from build123d import *

# Parameters (mm, degrees)
F0_W     = 82.55
F0_H     = 25.4
F1_DEPTH = 3.81
F2_W     = 2.54
F2_H     = 25.4
F3_DEPTH = 38.1
F4_R     = 7.62


with BuildPart() as f1:
    # F0 (on Top) → F1 (new body)
    with BuildSketch(Plane.XY):
        Rectangle(F0_W, F0_H)
    extrude(amount=F1_DEPTH)

    # F2 (on face) → F3 (join)
    with BuildSketch(Plane.XY.offset(3.81)):
        with Locations((-19.923125, 0)):
            Rectangle(F2_W, F2_H)
        with Locations((19.923125, 0)):
            Rectangle(F2_W, F2_H)
    extrude(amount=F3_DEPTH)

    # F4
    f4_edges = [f1.edges().sort_by_distance(p)[0] for p in [
        (-41.275, 12.7, 1.905),
        (-41.275, -12.7, 1.905),
        (41.275, 12.7, 1.905),
        (41.275, -12.7, 1.905),
        (-21.193125, 0, 3.81),
        (21.193125, 0, 3.81),
        (19.923125, 12.7, 41.91),
        (-19.923125, 12.7, 41.91),
        (-19.923125, -12.7, 41.91),
        (19.923125, -12.7, 41.91),
    ]]
    fillet(f4_edges, radius=F4_R)


solid = f1.part
Verification items for the finished model (mm, model axes). A direction names the side the tool comes from. Round coordinates to 2 decimals unless told otherwise and drop trailing zeros. Loops run counter-clockwise (first coordinate to the right, second up) from the corner with the lowest first, then second, coordinate; pieces in that order, holes last. Notation, with made-up numbers: (86.25, 49.5) - (96.25, 49.5) arc R18 cw to (96.25, 66.5) - close; hole circle Ø1 at (53.25, 8.5). An arc over 180 degrees is marked (long way). Answer in a Markdown table with one row per item. Add a question column.
Q1. Material ranges on line 1 (X direction, y = 2.25, z = 13); line 2 (Z direction, x = 12, y = -2.25); line 3 (X direction, y = -7.5, z = 6.5), recorded low to high.
Q2. Release check for a two-part mould opening along X. For faces 1 (the face through (-21.193, 0, 26)), 2 (the face through (18.653, 0, 23)), 3 (the face through (35, 0, 3.81)) record: pulls with the +X half, pulls with the -X half, needs draft (parallel to the pull), parting line crosses it, or undercut.
Q3. Section check B-B on y = -0.25. Enter the section's corners in (x, z) (3 decimals), plus the area to 3 significant figures.
Q4. Section check C-C on z = 39.5. Enter the section's corners in (x, y), plus the area to 3 significant figures.
Q5. Tool access check on faces 4 (the face through (-35, 0, 3.81)), 5 (the face through (0, 0, 3.81)), 6 (the face through (21.193, 0, 26)), 7 (the face through (-39.1, 10.41, 1.93)). Record the directions out of +Z, -Z, +X, -X, +Y, -Y that give a thin tool (end or side, any length) a straight path to the whole face; none if there is none.
Q6. Gauge pin test, flat ends, axial feed: pin 1 (3 mm diameter, centred on x = -9.5, y = 0.5, fed in from +Z); pin 2 (12 mm diameter, centred on x = -15, y = -7.5, fed in from +Z); pin 3 (7.5 mm diameter, centred on y = -6, z = 32.5, fed in from +X); pin 4 (6 mm diameter, centred on x = 24, z = 37, fed in from -Y). Record the tip position at first contact, or that the pin passes through.
Q7. Section check A-A on z = 17. Enter the section's corners in (x, y), plus the area to 3 significant figures.
Q8. Section check D-D on x = 11. Enter the section's corners in (y, z), plus the area to 3 significant figures.
Found:
| question | item | result |
|---|---|---|
| 1 | line 1 | x = -21.19 to -18.65, 18.65 to 21.19 |
| 1 | line 2 | z = 0 to 3.81 |
| 1 | line 3 | x = -23 to -18.65, 18.65 to 23 |
| 2 | face 1 | pulls with the -X half |
| 2 | face 2 | undercut |
| 2 | face 3 | needs draft |
| 3 | outline | (-41.275, 0) - (41.275, 0) - (41.275, 3.81) - (28.813, 3.81) arc R7.62 cw to (21.193, 11.43) - (21.193, 41.91) - (18.653, 41.91) - (18.653, 3.81) - (-18.653, 3.81) - (-18.653, 41.91) - (-21.193, 41.91) - (-21.193, 11.43) arc R7.62 cw to (-28.813, 3.81) - (-41.275, 3.81) - close |
| 3 | area | 533 mm² |
| 4 | outline | (-21.19, -10.64) - (-18.65, -10.64) - (-18.65, 10.64) - (-21.19, 10.64) - close; (18.65, -10.64) - (21.19, -10.64) - (21.19, 10.64) - (18.65, 10.64) - close |
| 4 | area | 108 mm² |
| 5 | face 4 | +Z, -X, +Y, -Y |
| 5 | face 5 | +Z, +Y, -Y |
| 5 | face 6 | +Z, +X, +Y, -Y |
| 5 | face 7 | +Z, -Z, -X, +Y |
| 6 | pin 1 | stops at z = 3.81 |
| 6 | pin 2 | stops at z = 41.91 |
| 6 | pin 3 | stops at x = 21.19 |
| 6 | pin 4 | stops at y = -12.52 |
| 7 | outline | (-21.19, -12.7) - (-18.65, -12.7) - (-18.65, 12.7) - (-21.19, 12.7) - close; (18.65, -12.7) - (21.19, -12.7) - (21.19, 12.7) - (18.65, 12.7) - close |
| 7 | area | 129 mm² |
| 8 | outline | (-12.7, 0) - (12.7, 0) - (12.7, 3.81) - (-12.7, 3.81) - close |
| 8 | area | 96.8 mm² |
